```python
from build123d import *

# Parameters (mm, degrees)
EXTRUDE_START        = 300
EXTRUDE_SKETCH_1_R   = 30
EXTRUDE_1_DEPTH      = 8
EXTRUDE_START_2      = 308
EXTRUDE_SKETCH_2_R   = 16
EXTRUDE_SKETCH_2_R_2 = 13.5
EXTRUDE_2_DEPTH      = 492


with BuildPart() as part:
    # Extrude sketch 1 → Extrude 1 (new body)
    with BuildSketch(Plane.XY.offset(EXTRUDE_START)):
        with Locations((860, 225)):
            Circle(EXTRUDE_SKETCH_1_R)
    extrude(amount=EXTRUDE_1_DEPTH)


with BuildPart() as body_2:
    # Extrude sketch 2 → Extrude 2 (new body)
    with BuildSketch(Plane.XY.offset(EXTRUDE_START_2)):
        with Locations((860, 225)):
            Circle(EXTRUDE_SKETCH_2_R)
        with Locations((860, 225)):
            Circle(EXTRUDE_SKETCH_2_R_2, mode=Mode.SUBTRACT)
    extrude(amount=EXTRUDE_2_DEPTH)


with BuildPart() as part_1:
    add(part.part)

    # Combine (weld / assembly of features): union body 2
    add(body_2.part)


solid = part_1.part
```
Build history of the part. All positions in model axes, mm. A direction names the side the tool comes from. Give positions to 0.01 mm unless a question says otherwise; leave off trailing zeros. Loops run counter-clockwise (first coordinate to the right, second up) from the corner with the lowest first, then second, coordinate; pieces in that order, holes last.
1) Band-saw the part on C-C on x = 860. List the corners of the cut face in (y, z).
Values follow:
outline: (195, 300) - (255, 300) - (255, 308) - (241, 308) - (241, 800) - (238.5, 800) - (238.5, 308) - (211.5, 308) - (211.5, 800) - (209, 800) - (209, 308) - (195, 308) - close
2) Band-saw the part on D-D on x = 884. List the corners of the cut face in (y, z).
Values follow:
outline: (207, 300) - (243, 300) - (243, 308) - (207, 308) - close
3) Two-plate mould, pull along Y, no slides. Class faces 1 (the face through (856.53, 209.38, 550.56)), 2 (the face through (853, 213, 800)), 3 (the face through (872.47, 219.83, 550.56)): released by +Y, released by -Y, zero draft, split by the parting line, or undercut.
Values follow:
face 1: split by the parting line
face 2: zero draft
face 3: undercut
4) Probe line 1 along Y through (x, z) = (861, 527); line 2 along Z through (x, y) = (874.5, 202.5); line 3 along Y through (x, z) = (865.5, 724). List the from-to ranges inside material, lowest first.
Values follow:
line 1: y = 209.03 to 211.54, 238.46 to 240.97
line 2: z = 300 to 308
line 3: y = 209.98 to 212.67, 237.33 to 240.02
5) Drop flat-ended pins along their axis: P1, Ø5, axis at y = 226, z = 392.5, coming from the -X side; P2, Ø24.5, axis at x = 860, y = 225, coming from the +Z side; P3, Ø3, axis at y = 233, z = 629.5, coming from the -X side. Give the stop position or say it passes through.
Values follow:
P1: stops at x = 844
P2: stops at z = 308
P3: stops at x = 845.38
6) Band-saw the part on B-B on z = 535. List the corners of the cut face in (x, y), then the cut area to 3 significant figures.
Values follow:
outline: circle Ø32 at (860, 225); hole circle Ø27 at (860, 225)
area: 232 mm2
7) Band-saw the part on A-A on y = 225. List the corners of the cut face in (x, z), then the cut area to 3 significant figures.
Values follow:
outline: (830, 300) - (890, 300) - (890, 308) - (876, 308) - (876, 800) - (873.5, 800) - (873.5, 308) - (846.5, 308) - (846.5, 800) - (844, 800) - (844, 308) - (830, 308) - close
area: 2,940 mm2
8) 3-axis set-ups, long thin cutter, end or side, ignore diameter. For faces 4 (the face through (860, 225, 308)), 5 (the face through (888.615, 234.011, 303.944)): which of +Z, -Z, +X, -X, +Y, -Y reach the whole face in a straight line?
Values follow:
face 4: +Z
face 5: +Z, -Z
